Check sheet for the modelled part. Datum: model origin and axes. Units: mm. A direction names the side the tool comes from. Give positions to 0.01 mm unless a question says otherwise; leave off trailing zeros. Write each loop counter-clockwise with the first axis right and the second up, starting at its lowest first coordinate (ties: lowest second). Pieces come first, ordered by that corner, then holes. Notation, with made-up numbers: (58.5, -38) -> (105.5, -38) arc R7 ccw to (105.5, -29) -> close; hole circle Ø4 at (86.25, -5). An arc over 180 degrees is marked (long way). Return JSON: item names as keys, results as strings.
from build123d import *

# Parameters (mm, degrees)
F1_DEPTH = 60.96


# Not quite as in the source:
# - a feature names something its author has since deleted; it is built from what else it names


with BuildPart() as f1:
    # F0 (on Front) → F1 (new body)
    with BuildSketch(Plane.XZ):
        with BuildLine():
            Line((-6.096, 685.5557686025), (-6.096, 75.9557686025))
            ThreePointArc((-6.096, 75.9557686025), (-74.9833545956, 13.5623203614), (-32.3157872997, -69.0081871317))
            Line((-32.3157872997, -69.0081871317), (-32.3157872997, -85.470431505))
            ThreePointArc((-32.3157872997, -85.470431505), (-34.8273647694, -187.19175255), (59.6940359728, -149.5189509783))
            Line((59.6940359728, -149.5189509783), (36.3618585551, -149.5189509783))
            ThreePointArc((36.3618585551, -149.5189509783), (-31.2215584924, -159.5238706884), (0, -98.7552030748))
            Line((0, -98.7552030748), (0, -76.2))
            ThreePointArc((0, -76.2), (76.1389176687, -3.0504452534), (6.096, 75.9557686025))
            Line((6.096, 75.9557686025), (6.096, 685.5557686025))
            Line((6.096, 685.5557686025), (-6.096, 685.5557686025))
        make_face()
    extrude(amount=F1_DEPTH)


solid = f1.part
(1) Cross-section at A-A on x = -22.5. Enter the section's corners in (y, z), then the cut area to 3 significant figures.
Reply:
{"outline": "(-60.96, -193.82) -> (0, -193.82) -> (0, -168.28) -> (-60.96, -168.28) -> close; (-60.96, -106.04) -> (0, -106.04) -> (0, 72.8) -> (-60.96, 72.8) -> close", "area": "12,500 mm^2"}
(2) Thickness scan on L1, parallel to Z at x = -2.5, y = -47.5; L2, parallel to Z at x = 0.5, y = -20; L3, parallel to X at y = -9.5, z = 540. Record the ranges inside material, lowest first.
Reply:
{"L1": "-198.07 to -175.48, -98.84 to 685.56", "L2": "-198.12 to -175.56, -76.2 to 685.56", "L3": "-6.1 to 6.1"}
(3) Depth check by flat-ended pin: pin 1 Ø10 at (x, y) = (-45, -37) entering from +Z; pin 2 Ø18.5 at (x, y) = (53, -34) entering from +Z; pin 3 Ø11.5 at (y, z) = (-39.5, -91) entering from +X. Enter the tip coordinate at first touch or a pass-through.
Reply:
{"pin 1": "z = 64.86", "pin 2": "z = 62.39", "pin 3": "x = 0"}
(4) Cross-section at C-C on z = -137.16. Enter the section's corners in (x, y).
Reply:
{"outline": "(-60.96, -60.96) -> (-38.4, -60.96) -> (-38.4, 0) -> (-60.96, 0) -> close"}
(5) Cross-section at B-B on y = -13. Enter the section's corners in (x, z).
Reply:
{"outline": "(-32.32, -85.47) arc R60.96 ccw (long way) to (59.69, -149.52) -> (36.36, -149.52) arc R38.4 cw (long way) to (0, -98.76) -> (0, -76.2) arc R76.2 ccw to (6.1, 75.96) -> (6.1, 685.56) -> (-6.1, 685.56) -> (-6.1, 75.96) arc R76.2 ccw to (-32.32, -69.01) -> close"}
(6) Cross-section at D-D on z = 628. Enter the section's corners in (x, y).
Reply:
{"outline": "(-6.1, -60.96) -> (6.1, -60.96) -> (6.1, 0) -> (-6.1, 0) -> close"}
(7) Set-up check for faces 4 (the flat face through (6.096, -30, 376)), 5 (the cylindrical face through (-74.72, -30.05, 14.94)), 6 (the flat face through (-6.096, -30, 385)), 7 (the flat face through (48, -30, -149.519)): record each of +Z, -Z, +X, -X, +Y, -Y from which the full face is reachable in a straight line by a thin tool's end or side.
Reply:
{"face 4": "+Z, +X, +Y, -Y", "face 5": "-X, +Y, -Y", "face 6": "+Z, -X, +Y, -Y", "face 7": "+X, +Y, -Y"}
(8) Release check for a two-part mould opening along Z. For faces 1 (the flat face through (0, -60.96, 82)), 2 (the flat face through (-32.316, -30, -77)), 3 (the cylindrical face through (76.056, -30.053, -4.681)) record: pulls with the +Z half, pulls with the -Z half, needs draft (parallel to the pull), parting line crosses it, or undercut.
Reply:
{"face 1": "needs draft", "face 2": "undercut", "face 3": "undercut"}
